Autodesk Inventor part; units mm, degrees
ref_plane "YZ Plane" through (0, 0, 0) normal (1, 0, 0) x (0, 1, 0)
ref_plane "XZ Plane" through (0, 0, 0) normal (0, 1, 0) x (-1, 0, 0)
ref_plane "XY Plane" through (0, 0, 0) normal (0, 0, 1) x (1, 0, 0)
sketch "Sketch1" plane through (0, 0, 0) normal (0, 0, 1) x (1, 0, 0)
  line L0 (0, 3.1673) -> (0, -2.4908)
  line L1 (-20.5368, 0) -> (25.7294, 0)
  line L2 (0, 0) -> (-9.8402, -9.8402)
  line L3 (0, 0) -> (13.9161, 0) construction
  line L4 (0, 0) -> (-23.2805, 23.2805)
  circle A0 centre (0, 0) radius 66.675
  point P0 (-16.1645, 16.1645)
  point P1 (-41.3092, 41.3092)
  point P2 (-41.3092, -41.3092)
  point P3 (-16.1645, -16.1645)
  point P4 (16.1645, 16.1645)
  point P5 (41.3092, 41.3092)
  point P6 (41.3092, -41.3092)
  point P7 (16.1645, -16.1645)
  point P8 (24.13, -47.9739)
  point P9 (24.13, 34.5761)
  point P10 (-24.13, 33.3061)
  point P11 (-24.13, -41.6239)
  dimension "d1" = 45
  dimension "d57" = 35.56
  dimension "d58" = 22.86
  dimension "d59" = 48.26
  dimension "d60" = 48.26
  dimension "d61" = 74.93
  dimension "d62" = 82.55
  dimension "d63" = 6.35
  dimension "d64" = 1.27
  dimension "d65" = 24.13
  dimension "d66" = 133.35
extrude "Extrusion1" add sketch "Sketch1" along normal blind 1.5875
hole "Hole1" at (-16.1645, 16.1645, 0) at (-41.3092, 41.3092, 0) at (-41.3092, -41.3092, 0) at (-16.1645, -16.1645, 0) at (41.3092, 41.3092, 0) at (16.1645, 16.1645, 0) at (16.1645, -16.1645, 0) at (41.3092, -41.3092, 0) direction (0, 0, 1) diameter 3.302 end through all
hole "Hole2" at (24.13, -47.9739, 0) at (24.13, 34.5761, 0) at (-24.13, 33.3061, 0) at (-24.13, -41.6239, 0) direction (0, 0, 1) diameter 2.159 end through all
properties part number "BaseTop"
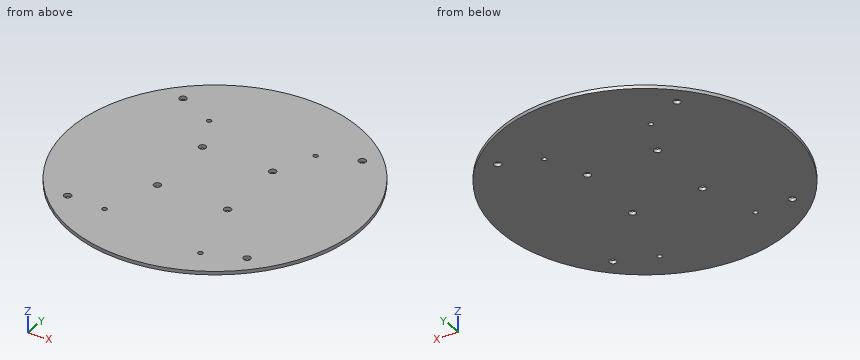
Geometry check sheet. Reference: the model listing, model coordinates, mm. Coordinates: 2 decimals unless noted, no trailing zeros. Order: outer loops, then holes, each group sorted by start corner. A loop starts at its lowest first (then second) coordinate and runs counter-clockwise, first axis right, second up. Notation, with made-up numbers: M 72,30 L 96,30 A13 ccw 96,55 Z; hole C 30.5,11 d6. An arc over 180 degrees is marked long. Answer as a JSON object with one key per item and string values.
Q1. Cross-section at C-C on x = -55.5. Record the cut outline in (y, z), and give its area (3 significant figures).
Results are:
{"outline": "M -36.95,0 L 36.95,0 L 36.95,1.59 L -36.95,1.59 Z", "area": "117 mm²"}
Q2. Scan lines: line 1 (X direction, y = -42, z = 1.15); line 2 (Y direction, x = 25, z = 0.9); line 3 (X direction, y = 41.5, z = 0.9). Record each from-to range of solid material in increasing order.
Results are:
{"line 1": "x = -51.78 to -42.81, -39.81 to -25.14, -23.12 to 39.81, 42.81 to 51.78", "line 2": "y = -61.81 to -48.61, -47.33 to 33.94, 35.22 to 61.81", "line 3": "x = -52.19 to -42.95, -39.67 to 39.67, 42.95 to 52.19"}
Q3. Depth check by flat-ended pin: pin 1 Ø1.7 at (x, y) = (-24.13, -41.62) entering from -Z. Enter the tip coordinate at first touch or a pass-through.
Results are:
{"pin 1": "passes through"}
Q4. Cross-section at A-A on z = 0.3. Give the number of separate pieces and of enclosed holes in the cut face, and give its area (3 significant figures).
Results are:
{"separate pieces": "1", "enclosed holes": "12", "area": "13,900 mm²"}
Q5. Cross-section at B-B on y = 24. Record the cut outline in (x, z).
Results are:
{"outline": "M -62.21,0 L 62.21,0 L 62.21,1.59 L -62.21,1.59 Z"}
